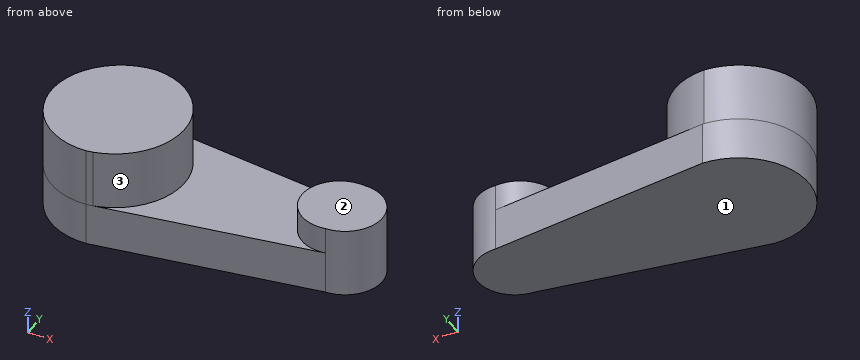
```python
from build123d import *

# Parameters (mm, degrees)
F2_DEPTH = 25.4
F4_DEPTH = 34.925
F6_DEPTH = 15.875


with BuildPart() as f2:
    # F0 (on Top) → F2 (new body)
    with BuildSketch(Plane.XY):
        with BuildLine():
            Line((133.35, 22.225), (0, 41.275))
            ThreePointArc((0, 41.275), (-41.703462, 0), (0, -41.275))
            Line((0, -41.275), (133.35, -22.225))
            ThreePointArc((133.35, -22.225), (155.575, 0), (133.35, 22.225))
        make_face()
    extrude(amount=F2_DEPTH)

    # F3 (on face) → F4 (join)
    with BuildSketch(Plane.XY.offset(25.4)):
        with BuildLine():
            ThreePointArc((-0.852523, 41.275), (-41.701261, -0.426261), (0, -41.275))
            Line((0, -41.275), (3.993336, -40.704523))
            ThreePointArc((3.993336, -40.704523), (37.493164, 2.408654), (-0.852523, 41.275))
        make_face()
    extrude(amount=F4_DEPTH)

    # F5 (on face) → F6 (join)
    with BuildSketch(Plane.XY.offset(25.4)):
        with BuildLine():
            ThreePointArc((133.35, -22.225), (155.575, 0), (133.35, 22.225))
            ThreePointArc((133.35, 22.225), (107.72436, 0), (133.35, -22.225))
        make_face()
    extrude(amount=F6_DEPTH)


solid = f2.part
```
Verification items for the finished model (mm, model axes). Face numbers are marked on the shaded views. A direction names the side the tool comes from. Give positions to 0.01 mm unless a question says otherwise; leave off trailing zeros. Loops run counter-clockwise (first coordinate to the right, second up) from the corner with the lowest first, then second, coordinate; pieces in that order, holes last.
1. Set-up check for the marked faces 1, 2 and 3: record each of +Z, -Z, +X, -X, +Y, -Y from which the full face is reachable in a straight line by a thin tool's end or side.
2. Section check D-D, the plane x = -12.5. Enter the section's corners in (y, z) (3 decimals), then the cut area to 3 significant figures.
3. Section check A-A, the plane y = 13. Enter the section's corners in (x, z) (3 decimals), then the cut area to 3 significant figures.
4. Go/stop test with flat-tipped pins: pin 1 Ø4 at (y, z) = (1, 40) entering from +X (3 decimals); pin 2 Ø12 at (y, z) = (7, 28) entering from -X; pin 3 Ø13.5 at (x, y) = (121.5, -10.5) entering from +Z (3 decimals). Record where each tip stops, or that it passes through.
5. Section check C-C, the plane z = 16. Enter the section's corners in (x, y) (3 decimals), then the cut area to 3 significant figures.
6. Thickness scan on line 1 (Z direction, x = 60.5, y = -15); line 2 (Y direction, x = -1, z = 26); line 3 (X direction, y = 16, z = 9). Record the ranges inside material, lowest first.
7. Section check B-B, the plane x = 113.5. Enter the section's corners in (y, z) (3 decimals).
Geometry says:
1. face 1: -Z, +X, -X, +Y, -Y
1. face 2: +Z, +X, +Y, -Y
1. face 3: +Z
2. outline: (-39.472, 0) - (39.472, 0) - (39.472, 60.325) - (-39.472, 60.325) - close
2. area: 4,760 mm2
3. outline: (-39.603, 0) - (151.376, 0) - (151.376, 41.275) - (111.871, 41.275) - (111.871, 25.4) - (35.461, 25.4) - (35.461, 60.325) - (-39.603, 60.325) - close
3. area: 8,100 mm2
4. pin 1: stops at x = 155.575
4. pin 2: stops at x = -41.69
4. pin 3: stops at z = 41.275
5. outline: (0, -41.275) - (133.35, -22.225) arc R22.225 ccw to (133.35, 22.225) - (0, 41.275) arc R41.277 ccw (long way) to start
5. area: 12,000 mm2
6. line 1: z = 0 to 25.4
6. line 2: y = -41.27 to 41.27
6. line 3: x = -38.48 to 148.78
7. outline: (-25.061, 0) - (25.061, 0) - (25.061, 25.4) - (15.032, 25.4) - (15.032, 41.275) - (-15.032, 41.275) - (-15.032, 25.4) - (-25.061, 25.4) - close
